Here's how the part is built. I have some questions about the finished solid (model axes, mm). Coordinates: 2 decimals unless noted, no trailing zeros. Order: outer loops, then holes, each group sorted by start corner. A loop starts at its lowest first (then second) coordinate and runs counter-clockwise, first axis right, second up. Notation, with made-up numbers: (59.25, 73) - (93.25, 73) arc R28 cw to (93.25, 99) - close; hole circle Ø7 at (13, 44). An arc over 180 degrees is marked (long way). Answer in a Markdown table with one row per item. Add a question column.
Item 1: Will these pins go through, and if not, where does the flat tip stop? pin 1 Ø3 at (x, y) = (0.5, 0) entering from +Z; pin 2 Ø4 at (x, z) = (0.5, -4.5) entering from -Y; pin 3 Ø2 at (y, z) = (-0.5, -4.5) entering from +X.
Item 2: I want a section at C-C (z = -4.25). Please give me the cut outline in (x, y), plus the area to 3 significant figures.
Item 3: If I drill on line 1 along Z through (x, y) = (1.5, 1.5); line 2 along Y through (x, z) = (0, -1.5); line 3 along X through (y, z) = (2.25, 0.5), over which ranges is the centre line in solid material (lowest first)? Write a range as from..to.
Item 4: I want a section at A-A (y = 0). Please give me the cut outline in (x, z).
Item 5: Thinking about a two-plate mould opening in X: for faces 1 (the flat face through (1, -1, 1)), 2 (the cylindrical face through (-0.108, 0.488, -2.859)), 3 (the flat face through (0, 0, 0.5)), which applies, +X half, -X half, draft (parallel to the pull), parting line (faces both ways), or undercut?
```python
from build123d import *

# Parameters (mm, degrees)
SKETCH1_R           = 3.5
BOSS_EXTRUDE1_DEPTH = 1
SKETCH2_R           = 0.5
BOSS_EXTRUDE2_DEPTH = 6
FILLET1_R           = 0.2
CUT_EXTRUDE1_DEPTH  = 0.5
CUT_EXTRUDE1_DRAFT  = -10
FILLET2_R           = 0.2


with BuildPart() as part:
    # Sketch1 → Boss-Extrude1 (new body)
    with BuildSketch(Plane.XY):
        Circle(SKETCH1_R)
    extrude(amount=BOSS_EXTRUDE1_DEPTH)

    # Sketch2 → Boss-Extrude2 (add)
    with BuildSketch(Plane(origin=(0, 0, 0), x_dir=(-1, 0, 0), z_dir=(0, 0, -1))):
        with Locations(Location((0, 0, 0), (0, 0, 180))):
            Circle(SKETCH2_R)
    extrude(amount=BOSS_EXTRUDE2_DEPTH)

    # Fillet1
    fillet1_edges = [part.edges().sort_by_distance(p)[0] for p in [
        (-3.5, 0, 1),
    ]]
    fillet(fillet1_edges, radius=FILLET1_R)


with BuildPart() as cut_extrude1_tool:
    # Sketch3 → Cut-Extrude1 (with draft: the straight prism first)
    with BuildSketch(Plane.XY.offset(1)):
        Polygon((-0.2, -0.2), (-0.2, -1.5), (0.2, -1.5), (0.2, -0.2), (1.5, -0.2), (1.5, 0.2), (0.2, 0.2), (0.2, 1.5), (-0.2, 1.5), (-0.2, 0.2), (-1.5, 0.2), (-1.5, -0.2), align=None)
    extrude(amount=-CUT_EXTRUDE1_DEPTH)
    # Cut-Extrude1: the draft: its side faces are tilted about the plane it starts from
    cut_extrude1_sides = [cut_extrude1_tool.faces().sort_by_distance(p)[0] for p in [
        (-0.2, -0.85, 0.75),
        (0, -1.5, 0.75),
        (0.2, -0.85, 0.75),
        (0.85, -0.2, 0.75),
        (1.5, 0, 0.75),
        (0.85, 0.2, 0.75),
        (0.2, 0.85, 0.75),
        (0, 1.5, 0.75),
        (-0.2, 0.85, 0.75),
        (-0.85, 0.2, 0.75),
        (-1.5, 0, 0.75),
        (-0.85, -0.2, 0.75),
    ]]
    draft(cut_extrude1_sides, Plane.XY.offset(1), CUT_EXTRUDE1_DRAFT)


with BuildPart() as part_1:
    add(part.part)

    # Cut-Extrude1: cut by cut_extrude1_tool
    add(cut_extrude1_tool.part, mode=Mode.SUBTRACT)

    # Fillet2
    fillet2_edges = [part_1.edges().sort_by_distance(p)[0] for p in [
        (-0.5, 0, -6),
    ]]
    fillet(fillet2_edges, radius=FILLET2_R)


solid = part_1.part
```
Values follow:
| question | item | result |
|---|---|---|
| 1 | pin 1 | stops at z = 1 |
| 1 | pin 2 | stops at y = -0.5 |
| 1 | pin 3 | stops at x = 0.5 |
| 2 | outline | circle Ø1 at (0, 0) |
| 2 | area | 0.785 mm^2 |
| 3 | line 1 | z = 0..1 |
| 3 | line 2 | y = -0.5..0.5 |
| 3 | line 3 | x = -2.68..2.68 |
| 4 | outline | (-3.5, 0) - (-0.5, 0) - (-0.5, -5.8) arc R0.2 ccw to (-0.3, -6) - (0.3, -6) arc R0.2 ccw to (0.5, -5.8) - (0.5, 0) - (3.5, 0) - (3.5, 0.8) arc R0.2 ccw to (3.3, 1) - (1.5, 1) - (1.41, 0.5) - (-1.41, 0.5) - (-1.5, 1) - (-3.3, 1) arc R0.2 ccw to (-3.5, 0.8) - close |
| 5 | face 1 | draft |
| 5 | face 2 | parting line |
| 5 | face 3 | undercut |
